```python
from build123d import *

# Parameters (mm, degrees)
ESBO_O1_W                = 90.06
ESBO_O1_H                = 30
RESSALTO_EXTRUS_O1_DEPTH = 5
ESBO_O2_W                = 70.2
ESBO_O2_H                = 24.3
CORTE_EXTRUS_O1_DEPTH    = 6
ESBO_O4_R                = 1.5
CORTE_EXTRUS_O2_DEPTH    = 10


with BuildPart() as part:
    # Esboço1 → Ressalto-extrusão1 (new body)
    with BuildSketch(Plane.XY):
        with Locations((19.809040323, 1.862332774)):
            Rectangle(ESBO_O1_W, ESBO_O1_H)
    extrude(amount=RESSALTO_EXTRUS_O1_DEPTH)

    # Esboço2 → Corte-extrusão1 (cut, through all)
    with BuildSketch(Plane(origin=(0, 0, 0), x_dir=(-1, 0, 0), z_dir=(0, 0, -1))):
        with Locations((-19.809040323, 1.712332774)):
            Rectangle(ESBO_O2_W, ESBO_O2_H)
    extrude(amount=-CORTE_EXTRUS_O1_DEPTH, mode=Mode.SUBTRACT)

    # Esboço4 → Corte-extrusão2 (cut)
    with BuildSketch(Plane(origin=(0, 0, 0), x_dir=(-1, 0, 0), z_dir=(0, 0, -1))):
        with Locations((22.720959677, 10.862332774)):
            Circle(ESBO_O4_R)
        with Locations((-62.339040323, 10.862332774)):
            Circle(ESBO_O4_R)
    extrude(amount=-CORTE_EXTRUS_O2_DEPTH, mode=Mode.SUBTRACT)


solid = part.part
```
Design review of the part built by this model. Coordinates are the model's own, in mm. A direction names the side the tool comes from. Coordinates: 2 decimals unless noted, no trailing zeros. Order: outer loops, then holes, each group sorted by start corner. A loop starts at its lowest first (then second) coordinate and runs counter-clockwise, first axis right, second up. Notation, with made-up numbers: (-36, -14.5) - (-26, -14.5) arc R34 cw to (-26, 15.5) - close; hole circle Ø1 at (25.25, 30). An arc over 180 degrees is marked (long way). Answer in a Markdown table with one row per item.
(1) The part is to be moulded in two halves that separate along Y. For faces 1 (the cylindrical face through (63.838, 10.928, 2.465)), 2 (the flat face through (20, -10.438, 2)), 3 (the flat face through (19, 16.862, 2)), 4 (the flat face through (19, -13.138, 2)), say which applies: released by +Y, released by -Y, zero draft, split by the parting line, or undercut.
Checked values:
| item | result |
|---|---|
| face 1 | undercut |
| face 2 | undercut |
| face 3 | released by +Y |
| face 4 | released by -Y |
(2) Consider section C-C on z = 3.4. State the section outline as (x, y) points, plus the area to 3 significant figures.
Checked values:
| item | result |
|---|---|
| outline | (-25.22, -13.14) - (64.84, -13.14) - (64.84, 16.86) - (-25.22, 16.86) - close; hole circle Ø3 at (-22.72, 10.86); hole (-15.29, -10.44) - (54.91, -10.44) - (54.91, 13.86) - (-15.29, 13.86) - close; hole circle Ø3 at (62.34, 10.86) |
| area | 982 mm^2 |
(3) Consider section B-B on x = 40.5. State the section outline as (y, z) points.
Checked values:
| item | result |
|---|---|
| outline | (-13.14, 0) - (-10.44, 0) - (-10.44, 5) - (-13.14, 5) - close; (13.86, 0) - (16.86, 0) - (16.86, 5) - (13.86, 5) - close |
(4) Consider section A-A on y = -5.5. State the section outline as (x, z) points.
Checked values:
| item | result |
|---|---|
| outline | (-25.22, 0) - (-15.29, 0) - (-15.29, 5) - (-25.22, 5) - close; (54.91, 0) - (64.84, 0) - (64.84, 5) - (54.91, 5) - close |
(5) Wall thickness on line 1 along Y through (x, z) = (-10.5, 3.2); line 2 along X through (y, z) = (12.5, 1.55); line 3 along X through (y, z) = (11, 2.2): over which ranges is each line inside the solid? List them lowest first. Write a range as from..to.
Checked values:
| item | result |
|---|---|
| line 1 | -13.14..-10.44, 13.86..16.86 |
| line 2 | -25.22..-15.29, 54.91..64.84 |
| line 3 | -25.22..-24.21, -21.23..-15.29, 54.91..60.85, 63.83..64.84 |
(6) For faces 5 (the flat face through (54.909, 2, 2)), 6 (the flat face through (64.839, 2, 2)), list the 3-axis set-ups (+Z, -Z, +X, -X, +Y, -Y) from which the entire face can be reached by the end or side of a thin tool; tool diameter is ignored.
Checked values:
| item | result |
|---|---|
| face 5 | +Z, -Z |
| face 6 | +Z, -Z, +X, +Y, -Y |
